from build123d import *

# Parameters (mm, degrees)
SKETCH_2_R      = 280
SKETCH_2_R_2    = 150
SKETCH_2_R_3    = 6.1
SKETCH_2_R_4    = 2.75
EXTRUDE_1_DEPTH = 10


with BuildPart() as part:
    # Эскиз2 → Бобышка-Вытянуть1 (new body)
    with BuildSketch(Plane(origin=(0, 0, 0), x_dir=(-1, 0, 0), z_dir=(0, 0, 1))):
        with Locations(Location((0, 0, 0), (0, 0, 180))):
            Circle(SKETCH_2_R)
        with Locations(Location((0, 0, 0), (0, 0, 180))):
            Circle(SKETCH_2_R_2, mode=Mode.SUBTRACT)
        with Locations(Location((-188, 0, 0), (0, 0, 180))):
            Circle(SKETCH_2_R_3, mode=Mode.SUBTRACT)
        with Locations(Location((-165.5, 0, 0), (0, 0, 180))):
            Circle(SKETCH_2_R_4, mode=Mode.SUBTRACT)
        with Locations(Location((-265, 0, 0), (0, 0, 180))):
            Circle(SKETCH_2_R_3, mode=Mode.SUBTRACT)
        with Locations(Location((-82.75, 143.327204326, 0), (0, 0, 180))):
            Circle(SKETCH_2_R_4, mode=Mode.SUBTRACT)
        with Locations(Location((82.75, 143.327204326, 0), (0, 0, 180))):
            Circle(SKETCH_2_R_4, mode=Mode.SUBTRACT)
        with Locations(Location((165.5, 0, 0), (0, 0, 180))):
            Circle(SKETCH_2_R_4, mode=Mode.SUBTRACT)
        with Locations(Location((82.75, -143.327204326, 0), (0, 0, 180))):
            Circle(SKETCH_2_R_4, mode=Mode.SUBTRACT)
        with Locations(Location((-82.75, -143.327204326, 0), (0, 0, 180))):
            Circle(SKETCH_2_R_4, mode=Mode.SUBTRACT)
        with Locations(Location((94, 162.812775911, 0), (0, 0, 180))):
            Circle(SKETCH_2_R_3, mode=Mode.SUBTRACT)
        with Locations(Location((94, -162.812775911, 0), (0, 0, 180))):
            Circle(SKETCH_2_R_3, mode=Mode.SUBTRACT)
        with Locations(Location((-132.5, 229.496732003, 0), (0, 0, 180))):
            Circle(SKETCH_2_R_3, mode=Mode.SUBTRACT)
        with Locations(Location((132.5, 229.496732003, 0), (0, 0, 180))):
            Circle(SKETCH_2_R_3, mode=Mode.SUBTRACT)
        with Locations(Location((265, 0, 0), (0, 0, 180))):
            Circle(SKETCH_2_R_3, mode=Mode.SUBTRACT)
        with Locations(Location((132.5, -229.496732003, 0), (0, 0, 180))):
            Circle(SKETCH_2_R_3, mode=Mode.SUBTRACT)
        with Locations(Location((-132.5, -229.496732003, 0), (0, 0, 180))):
            Circle(SKETCH_2_R_3, mode=Mode.SUBTRACT)
    extrude(amount=EXTRUDE_1_DEPTH)


solid = part.part
Source: CAD feature listing. Evaluate the final solid. Frame: model axes, mm. Round coordinates to 2 decimals unless told otherwise and drop trailing zeros. Loops run counter-clockwise (first coordinate to the right, second up) from the corner with the lowest first, then second, coordinate; pieces in that order, holes last. Notation, with made-up numbers: (64, 19) - (100, 19) arc R26 ccw to (100, 36) - close; hole circle Ø4 at (50.25, -10). An arc over 180 degrees is marked (long way). Write item = value, one per line. Start each with the question number.
Item 1: Material intervals for line 1 (Y direction, x = 132.5, z = 4.25); line 2 (Y direction, x = -82.75, z = 5.75); line 3 (Y direction, x = 0, z = 3), sorted ascending.
Item 2: Section query B-B on y = -58. Output: boundary loops of the cut face in (x, z), plus the area to 3 significant figures.
Item 3: First-contact query: pin 1 Ø6.5 at (x, y) = (-82.75, 143.33) entering from -Z; pin 2 Ø3 at (y, z) = (59, 7.5) entering from +X; pin 3 Ø6 at (x, z) = (125, 6) entering from -Y; pin 4 Ø1.5 at (y, z) = (-180, 7) entering from -X. Flat tips, straight axial feed; report the tip coordinate or a pass-through.
Item 4: Mould query, pull axis Y, two halves, no side actions, for faces 1 (the face through (-60.7, -273.34, 4.93)), 2 (the face through (121, -121, 10)), 3 (the face through (127.66, -233.21, 4.93)). Classes: released by +Y, released by -Y, zero draft, split by the parting line, or undercut.
Item 5: Section query C-C on z = 5.25. Count the separate pieces of the cut face and the enclosed holes in it, plus the area to 3 significant figures.
Item 6: Section query A-A on x = -29. Output: boundary loops of the cut face in (y, z).
Results list:
q1.line_1 = -246.67 to -235.6, -223.4 to -70.31, 70.31 to 223.4, 235.6 to 246.67
q1.line_2 = -267.49 to -146.08, -140.58 to -125.11, 125.11 to 140.58, 146.08 to 267.49
q1.line_3 = -280 to -150, 150 to 280
q2.outline = (-273.93, 0) - (-138.33, 0) - (-138.33, 10) - (-273.93, 10) - close; (138.33, 0) - (273.93, 0) - (273.93, 10) - (138.33, 10) - close
q2.area = 2,710 mm²
q3.pin_1 = 0
q3.pin_2 = 274.03
q3.pin_3 = -252.02
q3.pin_4 = -215.1
q4.face_1 = split by the parting line
q4.face_2 = zero draft
q4.face_3 = undercut
q5.separate_pieces = 1
q5.enclosed_holes = 16
q5.area = 174,000 mm²
q6.outline = (-278.49, 0) - (-147.17, 0) - (-147.17, 10) - (-278.49, 10) - close; (147.17, 0) - (278.49, 0) - (278.49, 10) - (147.17, 10) - close
